Autodesk Inventor part; units mm, degrees
ref_plane "YZ Plane" through (0, 0, 0) normal (1, 0, 0) x (0, 1, 0)
ref_plane "XZ Plane" through (0, 0, 0) normal (0, 1, 0) x (-1, 0, 0)
ref_plane "XY Plane" through (0, 0, 0) normal (0, 0, 1) x (1, 0, 0)
sketch "Sketch1" plane through (0, 0, 0) normal (1, 0, 0) x (0, 1, 0)
  line L0 (12.7, 6.35) -> (-12.7, 6.35) construction
  line L1 (-12.7, 6.35) -> (-12.7, -6.35)
  line L2 (-12.7, -6.35) -> (12.7, -6.35)
  line L3 (12.7, -6.35) -> (12.7, 6.35)
  line L4 (12.7, 6.35) -> (-12.7, -6.35) construction
  line L5 (-12.7, 6.35) -> (12.7, -6.35) construction
  circle A0 centre (0, 19.05) radius 6.35 construction
  line L6 (5.7876, 21.6626) -> (12.7, 6.35)
  line L7 (-5.7876, 21.6626) -> (-12.7, 6.35)
  arc A1 (5.7876, 21.6626) -> (-5.7876, 21.6626) centre (0, 19.05) ccw
  point P0 (0, 0)
  point P1 (0, 6.35)
  dimension "d0" = 25.4
  dimension "d1" = 12.7
  dimension "d2" = 12.7
  dimension "d3" = 12.7
extrude "Extrusion1" add sketch "Sketch1" along normal blind 19.05
hole "Hole1" at (0, 0, 19.05) direction (1, 0, 0) diameter 6.7564 end through all
sketch "Sketch2" plane through (0, -12.7, -6.35) normal (0, 0, -1) x (-1, 0, 0)
  line L0 (0, 25.4) -> (-19.05, 25.4) construction
  line L1 (0, 0) -> (-19.05, 0) construction
  line L2 (-9.525, 19.05) -> (-9.525, 6.35) construction
  line L3 (0, 0) -> (0, 25.4) construction
  point P0 (0, 12.7)
  point P1 (-9.525, 25.4)
  point P2 (-9.525, 0)
  point P3 (-9.525, 12.7)
  point P4 (0, 12.7)
  dimension "d13" = 12.7
hole "Hole2" at (9.525, 6.35, -6.35) at (9.525, -6.35, -6.35) direction (0, 0, 1) diameter 3.9624 depth 13.6144 tip angle 118
sketch "Sketch3" plane through (0, 12.7, 6.35) normal (0, 1, 0) x (1, 0, 0)
  line L0 (0, -15.3126) -> (0, -15.3126) construction
  line L1 (0, -15.3126) -> (19.05, -15.3126) construction
  line L2 (19.05, -15.3126) -> (19.05, -15.3126) construction
  line L3 (0, -15.3126) -> (19.05, -15.3126) construction
  line L4 (0, 0) -> (0, -15.3126) construction
  line L5 (0, -15.3126) -> (19.05, -15.3126) construction
  line L6 (19.05, 0) -> (19.05, -15.3126) construction
  line L7 (0, 0) -> (19.05, 0) construction
  line L8 (0, 12.7) -> (0, 0) construction
  line L9 (0, 0) -> (19.05, 0) construction
  line L10 (19.05, 12.7) -> (19.05, 0) construction
  line L11 (0, 12.7) -> (19.05, 12.7) construction
  line L12 (0, -19.05) -> (19.05, -19.05) construction
  line L13 (4.7625, -19.05) -> (14.2875, -19.05)
  line L14 (14.2875, -19.05) -> (14.2875, 0)
  line L15 (14.2875, 0) -> (4.7625, 0)
  line L16 (4.7625, 0) -> (4.7625, -19.05)
  point P0 (0, 6.35)
  point P1 (9.525, -19.05)
  point P2 (9.525, -19.05)
  dimension "d21" = 9.525
  dimension "d22" = 19.05
extrude "Extrusion2" cut sketch "Sketch3" against normal through all
properties part number "EL2-026-minusfillet" material "Aluminum 6061"
Geometry: final body of the model. Coordinates: model frame, mm. A direction names the side the tool comes from. Round coordinates to 2 decimals unless told otherwise and drop trailing zeros. Loops run counter-clockwise (first coordinate to the right, second up) from the corner with the lowest first, then second, coordinate; pieces in that order, holes last. Notation, with made-up numbers: M 4,4.25 L 28,4.25 A15 ccw 28,10.25 Z; hole C 29,-36 d3. An arc over 180 degrees is marked long. Put each result on its own line as item: value. Start each with the question number.
(1) Contact query for flat-ended pins moving along their axis: pin 1 Ø1 at (y, z) = (9, 16.5) entering from -X; pin 2 Ø4 at (x, z) = (12.5, 10) entering from -Y; pin 3 Ø3 at (x, y) = (8, -3.5) entering from +Z; pin 4 Ø4 at (x, z) = (6.5, 17.5) entering from -Y. Output: stop coordinate, or through.
(2) Section query A-A (y = -7.5). Return loops of the section in (x, z), then the cut area to 3 significant figures.
(3) Material intervals for line 1 along Z through (x, y) = (1, 0); line 2 along X through (y, z) = (5, 21); line 3 along X through (y, z) = (6.35, -3.25), sorted ascending. Write a range as [from, to].
(4) Section query C-C (z = 11.5). Return loops of the section in (x, y), then the cut area to 3 significant figures.
(5) Set-up query: faces 1 (the face through (2.415, 1.294, 22.171)), 2 (the face through (4.762, 0, 14)). Return all of +Z, -Z, +X, -X, +Y, -Y with unobstructed straight access to the full face (end or side cutting, diameter ignored); none if empty.
(6) Section query D-D (z = 19.05). Return loops of the section in (x, y), then the cut area to 3 significant figures.
(7) Section query B-B (y = 0). Return loops of the section in (x, z).
(8) Draft query along Y for faces 3 (the face through (9, 12.7, 0)), 4 (the face through (8.93, 8.24, 0.09)), 5 (the face through (16.6, -9.2, 14.1)). Return one class per face: +Y half, -Y half, draft (parallel to the pull), parting line (faces both ways), or undercut.
Findings below:
1. pin 1: passes through
1. pin 2: stops at y = -11.46
1. pin 3: stops at z = 6.35
1. pin 4: stops at y = -8.11
2. outline: M 0,-6.35 L 7.91,-6.35 L 7.91,6.35 L 4.76,6.35 L 4.76,17.87 L 0,17.87 Z; M 11.14,-6.35 L 19.05,-6.35 L 19.05,17.87 L 14.29,17.87 L 14.29,6.35 L 11.14,6.35 Z
2. area: 311 mm2
3. line 1: z = [-6.35, 15.67], [22.43, 25.4]
3. line 2: x = [0, 4.76], [14.29, 19.05]
3. line 3: x = [0, 7.54], [11.51, 19.05]
4. outline: M 0,-10.38 L 4.76,-10.38 L 4.76,10.38 L 0,10.38 Z; M 14.29,-10.38 L 19.05,-10.38 L 19.05,10.38 L 14.29,10.38 Z
4. area: 198 mm2
5. face 1: +X, -X
5. face 2: +Z, +Y, -Y
6. outline: M 0,-6.97 L 4.76,-6.97 L 4.76,-3.38 L 0,-3.38 Z; M 0,3.38 L 4.76,3.38 L 4.76,6.97 L 0,6.97 Z; M 14.29,-6.97 L 19.05,-6.97 L 19.05,-3.38 L 14.29,-3.38 Z; M 14.29,3.38 L 19.05,3.38 L 19.05,6.97 L 14.29,6.97 Z
6. area: 68.4 mm2
7. outline: M 0,-6.35 L 19.05,-6.35 L 19.05,15.67 L 14.29,15.67 L 14.29,6.35 L 4.76,6.35 L 4.76,15.67 L 0,15.67 Z; M 0,22.43 L 4.76,22.43 L 4.76,25.4 L 0,25.4 Z; M 14.29,22.43 L 19.05,22.43 L 19.05,25.4 L 14.29,25.4 Z
8. face 3: +Y half
8. face 4: undercut
8. face 5: -Y half
